```python
from build123d import *

# Parameters (mm, degrees)
F0_R     = 150
F0_R_2   = 123.825
F1_DEPTH = 9
F2_R     = 2.5
F3_DEPTH = 25.4


with BuildPart() as f1:
    # F0 (on Top) → F1 (new body)
    with BuildSketch(Plane.XY):
        Circle(F0_R)
        Circle(F0_R_2, mode=Mode.SUBTRACT)
    extrude(amount=F1_DEPTH)

    # F2 (on face) → F3 (cut)
    with BuildSketch(Plane.XY.offset(9)):
        with Locations((-94.292689, -94.292689)):
            Circle(F2_R)
        with Locations((93.755721, -94.829657)):
            Circle(F2_R)
        with Locations((94.292689, 93.218753)):
            Circle(F2_R)
        with Locations((-93.755721, 93.755721)):
            Circle(F2_R)
        with Locations((0, 143.131807)):
            Circle(F2_R)
        with Locations((123.955781, 71.565904)):
            Circle(F2_R)
        with Locations((123.955781, -71.565904)):
            Circle(F2_R)
        with Locations((0, -143.131807)):
            Circle(F2_R)
        with Locations((-123.955782, -71.565903)):
            Circle(F2_R)
        with Locations((-123.955781, 71.565904)):
            Circle(F2_R)
    extrude(amount=-F3_DEPTH, mode=Mode.SUBTRACT)


solid = f1.part
```
Build history of the part. All positions in model axes, mm. Coordinates: 2 decimals unless noted, no trailing zeros. Order: outer loops, then holes, each group sorted by start corner. A loop starts at its lowest first (then second) coordinate and runs counter-clockwise, first axis right, second up. Notation, with made-up numbers: (56, 4) -> (83, 4) arc R34 ccw to (83, 36) -> close; hole circle Ø7 at (80.5, -38.75). An arc over 180 degrees is marked (long way). Answer in a Markdown table with one row per item. Add a question column.
Q1. Drop flat-ended pins along their axis: pin 1 (1.5 mm diameter, centred on x = 18.5, z = 1, fed in from +Y); pin 2 (3 mm diameter, centred on x = 0, y = 143.13, fed in from -Z); pin 3 (4 mm diameter, centred on x = 33.5, z = 3.5, fed in from +Y); pin 4 (4 mm diameter, centred on y = 63, z = 3, fed in from -X). Give the stop position or say it passes through.
Q2. Band-saw the part on B-B, the plane x = 62.5. List the corners of the cut face in (y, z).
Q3. Wall check: line 1 along Y through (x, z) = (0, 3) (3 decimals); line 2 along X through (y, z) = (15.5, 5.5); line 3 along X through (y, z) = (-95, 1.5). Give the ranges that are in metal, low to high. Write a range as [from, to].
Q4. Band-saw the part on A-A, the plane y = 0. List the corners of the cut face in (x, z) (3 decimals), then the cut area to 3 significant figures.
Q5. Mould opens along Y. For faces 1 (the face through (-19.527, 148.724, 4.437)), 2 (the face through (-23, 123, 0)), 3 (the face through (-26.84, -120.88, 4.44)) say: +Y half, -Y half, draft (parallel to the pull), parting line (faces both ways), or undercut.
Q6. Band-saw the part on C-C, the plane z = 3.5. Give the number of separate pieces and of enclosed holes in the cut face, then the cut area to 3 significant figures.
Answers follow:
| question | item | result |
|---|---|---|
| 1 | pin 1 | y = 148.95 |
| 1 | pin 2 | through |
| 1 | pin 3 | y = 146.66 |
| 1 | pin 4 | x = -137.04 |
| 2 | outline | (-136.36, 0) -> (-106.89, 0) -> (-106.89, 9) -> (-136.36, 9) -> close; (106.89, 0) -> (136.36, 0) -> (136.36, 9) -> (106.89, 9) -> close |
| 3 | line 1 | [-150, -145.632], [-140.632, -123.825], [123.825, 140.632], [145.632, 150] |
| 3 | line 2 | [-149.2, -122.85], [122.85, 149.2] |
| 3 | line 3 | [-116.08, -96.69], [-91.89, -79.42], [79.42, 91.26], [96.25, 116.08] |
| 4 | outline | (-150, 0) -> (-123.825, 0) -> (-123.825, 9) -> (-150, 9) -> close; (123.825, 0) -> (150, 0) -> (150, 9) -> (123.825, 9) -> close |
| 4 | area | 471 mm^2 |
| 5 | face 1 | parting line |
| 5 | face 2 | draft |
| 5 | face 3 | undercut |
| 6 | separate pieces | 1 |
| 6 | enclosed holes | 11 |
| 6 | area | 22,300 mm^2 |
